Autodesk Fusion 360 part; units mm, degrees
sketch "Sketch6" plane through (0, 0, 0) normal (0, 0, 1) x (1, 0, 0)
  line L0 (-20, -140) -> (430.8, -140)
  line L1 (430.8, -140) -> (430.8, -294.5)
  line L2 (430.8, -294.5) -> (-20, -294.5)
  line L3 (-20, -294.5) -> (-20, -140)
  dimension "d40" = 450.8
  dimension "d41" = 154.5
extrude "Extrude8" add sketch "Sketch6" along normal blind 1
sketch "Sketch7" plane through (0, 0, 1) normal (0, 0, 1) x (-1, 0, 0)
  line L0 (20, 294.5) -> (-430.8, 294.5)
  line L1 (-430.8, 294.5) -> (-430.8, 140)
  line L2 (-430.8, 140) -> (20, 140)
  line L3 (20, 140) -> (20, 294.5)
  line L4 (-358.09, 140) -> (-378.09, 140)
  line L5 (-378.09, 140) -> (-378.09, 184)
  line L6 (-378.09, 184) -> (-358.09, 184)
  line L7 (-358.09, 184) -> (-358.09, 140)
  line L8 (-378.09, 184) -> (-419.8, 184)
  line L9 (-419.8, 184) -> (-419.8, 149.5)
  line L10 (-419.8, 149.5) -> (-378.09, 149.5)
  line L11 (-378.09, 149.5) -> (-378.09, 184)
  line L12 (10.5, 149.5) -> (-343.5, 149.5)
  line L13 (-343.5, 149.5) -> (-343.5, 284)
  line L14 (-343.5, 284) -> (10.5, 284)
  line L15 (10.5, 284) -> (10.5, 149.5)
  line L16 (-356.3, 220) -> (-420.3, 220)
  line L17 (-420.3, 220) -> (-420.3, 284)
  line L18 (-420.3, 284) -> (-356.3, 284)
  line L19 (-356.3, 284) -> (-356.3, 220)
  circle A0 centre (-426.8, 144) radius 1.1
  circle A1 centre (-426.8, 290.5) radius 1.1
  circle A2 centre (16, 290.5) radius 1.1
  circle A3 centre (16, 144) radius 1.1
  dimension "d46" = 20
  dimension "d47" = 44
  dimension "d48" = 52.71
  dimension "d51" = 41.71
  dimension "d52" = 34.5
  dimension "d55" = 354
  dimension "d56" = 134.5
  dimension "d57" = 9.5
  dimension "d58" = 9.5
  dimension "d59" = 64
  dimension "d60" = 64
  dimension "d61" = 10.5
  dimension "d62" = 10.5
  dimension "d67" = 2.2
  dimension "d68" = 2.2
  dimension "d69" = 2.2
  dimension "d70" = 2.2
  dimension "d71" = 4
  dimension "d72" = 4
  dimension "d73" = 4
  dimension "d74" = 4
  dimension "d75" = 4
  dimension "d76" = 4
  dimension "d77" = 4
  dimension "d78" = 4
extrude "Extrude9" cut sketch "Sketch7" against normal blind 1 contours L2 L4 L5 L6 L7 L11
extrude "Extrude10" cut sketch "Sketch7" against normal blind 1 contours L5 L8 L9 L10 L11
extrude "Extrude11" cut sketch "Sketch7" against normal blind 1 contours L12 L13 L14 L15 | L16 L17 L18 L19
fillet "Fillet6" radius 6 4 edges at (-20, -294.5, 0.5) (-20, -140, 0.5) (430.8, -140, 0.5) (430.8, -294.5, 0.5)
extrude "Extrude12" cut sketch "Sketch7" against normal blind 1 contours A0 | A1 | A2 | A3
equation "d51 = 52.210 mm - 10.50 mm"
equation "d52 = 44 mm - 9.5 mm"
Model file for the job. Use its own axes, mm. Give positions to 0.01 mm unless a question says otherwise; leave off trailing zeros. Loops run counter-clockwise (first coordinate to the right, second up) from the corner with the lowest first, then second, coordinate; pieces in that order, holes last.
1) Saw through at D-D (x = 382). Write the cut outline in (y, z), plus the area to 3 significant figures.
2) Wall check: line 1 (X direction, y = -160.5, z = 0.25); line 2 (X direction, y = -280, z = 0.8); line 3 (Y direction, x = 40, z = 0.85). Give the ranges that are in metal, low to high.
3) Saw through at B-B (y = -215). Write the cut outline in (x, z).
4) Saw through at C-C (z = 0.8). Write the cut outline in (x, y), plus the area to 3 significant figures.
5) Saw through at A-A (x = 112). Write the cut outline in (y, z), plus the area to 3 significant figures.
Answer block:
1. outline: (-294.5, 0) - (-284, 0) - (-284, 1) - (-294.5, 1) - close; (-220, 0) - (-184, 0) - (-184, 1) - (-220, 1) - close; (-149.5, 0) - (-140, 0) - (-140, 1) - (-149.5, 1) - close
1. area: 56.0 mm2
2. line 1: x = -20 to -10.5, 343.5 to 358.09, 419.8 to 430.8
2. line 2: x = -20 to -10.5, 343.5 to 356.3, 420.3 to 430.8
2. line 3: y = -294.5 to -284, -149.5 to -140
3. outline: (-20, 0) - (-10.5, 0) - (-10.5, 1) - (-20, 1) - close; (343.5, 0) - (430.8, 0) - (430.8, 1) - (343.5, 1) - close
4. outline: (-20, -288.5) arc R6 ccw to (-14, -294.5) - (424.8, -294.5) arc R6 ccw to (430.8, -288.5) - (430.8, -146) arc R6 ccw to (424.8, -140) - (378.09, -140) - (378.09, -149.5) - (419.8, -149.5) - (419.8, -184) - (358.09, -184) - (358.09, -140) - (-14, -140) arc R6 ccw to (-20, -146) - close; hole circle Ø2.2 at (-16, -290.5); hole circle Ø2.2 at (-16, -144); hole (-10.5, -284) - (343.5, -284) - (343.5, -149.5) - (-10.5, -149.5) - close; hole (356.3, -284) - (420.3, -284) - (420.3, -220) - (356.3, -220) - close; hole circle Ø2.2 at (426.8, -290.5); hole circle Ø2.2 at (426.8, -144)
4. area: 15,600 mm2
5. outline: (-294.5, 0) - (-284, 0) - (-284, 1) - (-294.5, 1) - close; (-149.5, 0) - (-140, 0) - (-140, 1) - (-149.5, 1) - close
5. area: 20.0 mm2
